Build history of the part. All positions in model axes, mm. Face numbers are marked on the shaded views. Coordinates: 2 decimals unless noted, no trailing zeros. Write each loop counter-clockwise with the first axis right and the second up, starting at its lowest first coordinate (ties: lowest second). Pieces come first, ordered by that corner, then holes. Notation, with made-up numbers: M -29.5,-11.5 L 12.5,-11.5 A21 cw 12.5,19.5 Z; hole C 25.5,-5 d8. An arc over 180 degrees is marked long. Use CSV: the item, a comma, the result in double quotes. Start each with the question number.
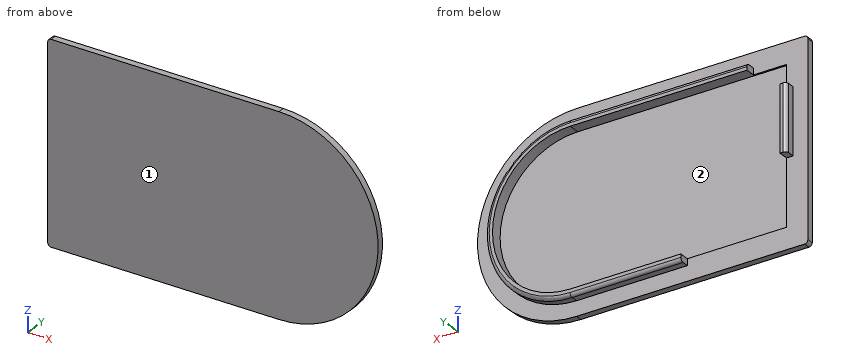
```python
from build123d import *

# Parameters (mm, degrees)
BOSS_EXTRUDE1_DEPTH = 3
BOSS_EXTRUDE2_START = 2
BOSS_EXTRUDE2_DEPTH = 2
CUT_EXTRUDE1_DEPTH  = 3.5
FILLET1_R           = 1
SKETCH5_W           = 12
SKETCH5_H           = 9
SKETCH5_W_2         = 32
SKETCH5_H_2         = 22
CUT_EXTRUDE4_DEPTH  = 3
FILLET8_R           = 1
FILLET9_R           = 1


with BuildPart() as part:
    # Sketch1 → Boss-Extrude1 (new body)
    with BuildSketch(Plane(origin=(0, 0, 0), x_dir=(1, 0, 0), z_dir=(0, 1, 0))):
        with BuildLine():
            Line((-65.5, -25.5), (0, -25.5))
            ThreePointArc((0, -25.5), (25.5, 0), (0, 25.5))
            Line((0, 25.5), (-65.5, 25.5))
            Line((-65.5, 25.5), (-65.5, -25.5))
        make_face()
    extrude(amount=BOSS_EXTRUDE1_DEPTH)

    # Sketch2 → Boss-Extrude2 (add)
    # profile 1 of 2: a face of its own
    with BuildSketch(Plane.XZ.offset(BOSS_EXTRUDE2_START)):
        with BuildLine():
            Line((-70, -30), (0, -30))
            ThreePointArc((0, -30), (30, 0), (0, 30))
            Line((0, 30), (-70, 30))
            Line((-70, 30), (-70, -30))
        make_face()
        with BuildLine():
            Line((0, 25.5), (-65.5, 25.5))
            Line((-65.5, 25.5), (-65.5, -25.5))
            Line((-65.5, -25.5), (0, -25.5))
            ThreePointArc((0, -25.5), (25.5, 0), (0, 25.5))
        make_face(mode=Mode.SUBTRACT)
    # profile 2 of 2: a face of its own
    with BuildSketch(Plane.XZ.offset(BOSS_EXTRUDE2_START)):
        with BuildLine():
            ThreePointArc((0, -25.5), (25.5, 0), (0, 25.5))
            Line((0, 25.5), (-65.5, 25.5))
            Line((-65.5, 25.5), (-65.5, -25.5))
            Line((-65.5, -25.5), (0, -25.5))
        make_face()
    extrude(amount=-BOSS_EXTRUDE2_DEPTH)

    # Sketch4 → Cut-Extrude1 (cut)
    with BuildSketch(Plane(origin=(0, 3, 0), x_dir=(1, 0, 0), z_dir=(0, 1, 0))):
        with BuildLine():
            Line((-63.5, -23.5), (0, -23.5))
            ThreePointArc((0, -23.5), (23.5, 0), (0, 23.5))
            Line((0, 23.5), (-63.5, 23.5))
            Line((-63.5, 23.5), (-63.5, -23.5))
        make_face()
    extrude(amount=-CUT_EXTRUDE1_DEPTH, mode=Mode.SUBTRACT)

    # Fillet1
    fillet1_edges = [part.edges().sort_by_distance(p)[0] for p in [
        (-70, -1, -30),
        (-70, -1, 30),
    ]]
    fillet(fillet1_edges, radius=FILLET1_R)

    # Sketch5 → Cut-Extrude4 (cut)
    with BuildSketch(Plane(origin=(0, 3, 0), x_dir=(1, 0, 0), z_dir=(0, 1, 0))):
        with Locations((-59.5, -21)):
            Rectangle(SKETCH5_W, SKETCH5_H)
        with Locations((-49.5, 14.5)):
            Rectangle(SKETCH5_W_2, SKETCH5_H_2)
    extrude(amount=-CUT_EXTRUDE4_DEPTH, mode=Mode.SUBTRACT)

    # Fillet8
    fillet8_edges = [part.edges().sort_by_distance(p)[0] for p in [
        (-65.5, 3, 6.5),
    ]]
    fillet(fillet8_edges, radius=FILLET8_R)

    # Fillet9
    fillet9_edges = [part.edges().sort_by_distance(p)[0] for p in [
        (25.5, 3, 0),
        (-16.75, 3, -25.5),
        (-26.75, 3, 25.5),
    ]]
    fillet(fillet9_edges, radius=FILLET9_R)


solid = part.part
```
1. Slice it at D-D (x = -38). List the corners of the cut face in (y, z), and give its area (3 significant figures).
2. Slice it at B-B (x = -62.5). List the corners of the cut face in (y, z).
3. Slice it at C-C (z = 0). List the corners of the cut face in (x, y), and give its area (3 significant figures).
4. Flat gauge pins, fed straight in: pin 1 (1.6 mm diameter, centred on y = 2, z = -25, fed in from -X); pin 2 (3 mm diameter, centred on y = 2, z = -10.5, fed in from +X); pin 3 (6 mm diameter, centred on x = -6, z = 0, fed in from +Y). Where does each tip first touch, or does it go through?
5. Drill centre lines: line 1 along Z through (x, y) = (-18, -0.25); line 2 along Z through (x, y) = (-31, 0.2); line 3 along X through (y, z) = (0.85, 0). Where is each one in solid material? Low to high. Write a range as from..to.
6. Slice it at A-A (y = 1). List the corners of the cut face in (x, z), and give its area (3 significant figures).
7. Pull direction Z, two halves, no side cores. Call the marked faces 1 and 2: pulls with the +Z half, pulls with the -Z half, needs draft (parallel to the pull), parting line crosses it, or undercut.
Established:
1,outline,"M -2,-30 L 0,-30 L 0,-23.5 L -0.5,-23.5 L -0.5,23.5 L 3,23.5 L 3,24.5 A1 ccw 2,25.5 L 0,25.5 L 0,30 L -2,30 Z"
1,area,"102 mm2"
2,outline,"M -2,-30 L 0,-30 L 0,-23.5 L -0.5,-23.5 L -0.5,23.5 L 0,23.5 L 0,30 L -2,30 Z"
3,outline,"M -70,-2 L 30,-2 L 30,0 L 25.5,0 L 25.5,2 A1 ccw 24.5,3 L 23.5,3 L 23.5,-0.5 L -63.5,-0.5 L -63.5,3 L -64.5,3 A1 ccw -65.5,2 L -65.5,0 L -70,0 Z"
3,area,"168 mm2"
4,pin 1,"stops at x = -33.5"
4,pin 2,"stops at x = 23.86"
4,pin 3,"stops at y = -0.5"
5,line 1,"z = -30..-23.5, 23.5..30"
5,line 2,"z = -25.5..-23.5, 23.5..25.5"
5,line 3,"x = -65.5..-63.5, 23.5..25.5"
6,outline,"M -65.5,-3.5 L -63.5,-3.5 L -63.5,16.5 L -65.5,16.5 Z; M -53.5,23.5 L 0,23.5 A23.5 cw 0,-23.5 L -33.5,-23.5 L -33.5,-25.5 L 0,-25.5 A25.5 ccw 0,25.5 L -53.5,25.5 Z"
6,area,"368 mm2"
7,face 1,"needs draft"
7,face 2,"undercut"
